The listing builds one solid part. Answer for the finished solid, in the listing's coordinates (mm). Face numbers are marked on the shaded views. A direction names the side the tool comes from. Round coordinates to 2 decimals unless told otherwise and drop trailing zeros. Order: outer loops, then holes, each group sorted by start corner. A loop starts at its lowest first (then second) coordinate and runs counter-clockwise, first axis right, second up. Notation, with made-up numbers: (-23.75, -12.75) - (27.25, -12.75) arc R12 ccw to (27.25, 6.25) - close; hole circle Ø11 at (-21.75, 56.25). An arc over 180 degrees is marked (long way). Write item = value, one per line.
from build123d import *

# Parameters (mm, degrees)
SKETCH143_W     = 21.769744
SKETCH143_H     = 51.763626
SKETCH143_R     = 2.629917
SKETCH143_R_2   = 2.549682
PAD053_DEPTH    = 5
SKETCH142_W     = 4.89418
SKETCH142_H     = 20.822479
PAD052_DEPTH    = 10
SKETCH141_R     = 3
POCKET084_DEPTH = 5


with BuildPart() as part:
    # Sketch143 → Pad053 (new body)
    with BuildSketch(Plane(origin=(195, 362, 200), x_dir=(1, 0, 0), z_dir=(0, -1, 0))):
        with Locations((1.846756, 20.929451)):
            Rectangle(SKETCH143_W, SKETCH143_H)
        with Locations((-2.70076, 40.56488)):
            Circle(SKETCH143_R, mode=Mode.SUBTRACT)
        with Locations((-2.789749, 0.699631)):
            Circle(SKETCH143_R_2, mode=Mode.SUBTRACT)
    extrude(amount=PAD053_DEPTH)

    # Sketch142 → Pad052 (new body)
    with BuildSketch(Plane(origin=(195, 357, 200), x_dir=(1, 0, 0), z_dir=(0, -1, 0))):
        with Locations((10.193657, 20.639526)):
            Rectangle(SKETCH142_W, SKETCH142_H)
    extrude(amount=PAD052_DEPTH)

    # Sketch141 → Pocket084 (cut)
    with BuildSketch(Plane(origin=(202.746567, 362, 200), x_dir=(0, 0, -1), z_dir=(-1, 0, 0))):
        with Locations((-20.563114, 10.481458)):
            Circle(SKETCH141_R)
    extrude(amount=-POCKET084_DEPTH, mode=Mode.SUBTRACT)


solid = part.part
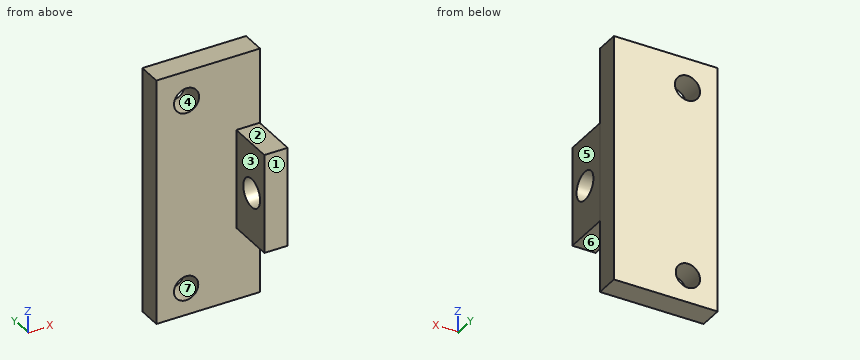
Q1. Section D-D on z = 240 is taken. Determine the outline of the cut face in (x, y), then the cut area to 3 significant figures.
Model answer:
outline = (185.96, 357) - (189.73, 357) - (189.73, 362) - (185.96, 362) - close; (194.87, 357) - (207.73, 357) - (207.73, 362) - (194.87, 362) - close
area = 83.2 mm^2
Q2. Section A-A on y = 352 is taken. Determine the outline of the cut face in (x, z), then the cut area to 3 significant figures.
Model answer:
outline = (202.75, 210.23) - (207.64, 210.23) - (207.64, 217.6) - (202.75, 217.6) - close; (202.75, 223.52) - (207.64, 223.52) - (207.64, 231.05) - (202.75, 231.05) - close
area = 72.9 mm^2
Q3. Section B-B on z = 212 is taken. Determine the outline of the cut face in (x, y), then the cut area to 3 significant figures.
Model answer:
outline = (185.96, 357) - (202.75, 357) - (202.75, 347) - (207.64, 347) - (207.64, 357) - (207.73, 357) - (207.73, 362) - (185.96, 362) - close
area = 158 mm^2
Q4. Section C-C on x = 203.75 is taken. Determine the outline of the cut face in (y, z).
Model answer:
outline = (347, 210.23) - (357, 210.23) - (357, 195.05) - (362, 195.05) - (362, 246.81) - (357, 246.81) - (357, 231.05) - (347, 231.05) - close; hole circle Ø6 at (351.52, 220.56)
Q5. Find the intervals of material crossed by line 1 (X direction, y = 356.75, z = 230.5); line 2 (Y direction, x = 206.25, z = 233.5); line 3 (Z direction, x = 192.75, y = 358.25), in increasing order. Write a range as from..to.
Model answer:
line_1 = 202.75..207.64
line_2 = 357..362
line_3 = 195.05..198.21, 203.19..237.97, 243.16..246.81
Q6. Flat-ended cylindrical pins translate along their axes: P1, Ø7, axis at y = 351.52, z = 220.56, coming from the +X side; P2, Ø2.5, axis at x = 206.5, y = 351.5, coming from the +Z side; P3, Ø5, axis at x = 202, y = 353, coming from the -Z side. Find the tip coordinate at first contact, or state that the pin passes through.
Model answer:
P1 = 207.64
P2 = 231.05
P3 = 210.23
Q7. For the marked faces 1, 2 and 3, determine the directions among +Z, -Z, +X, -X, +Y, -Y from which every point of the face is accessible in a straight line to the end or side of a thin tool.
Model answer:
face_1 = +Z, -Z, +X, -X, -Y
face_2 = +Z, +X, -X, -Y
face_3 = +Z, -Z, -X, -Y
Q8. Determine the mould class of the marked faces 4, 5, 6 and 7 for opening direction Z: released by +Z, released by -Z, zero draft, split by the parting line, or undercut.
Model answer:
face_4 = undercut
face_5 = zero draft
face_6 = released by -Z
face_7 = undercut
